Read the model definition and answer for the solid it produces. Units are mm, in the model's axes. Face numbers are marked on the shaded views. Coordinates: 2 decimals unless noted, no trailing zeros. Write each loop counter-clockwise with the first axis right and the second up, starting at its lowest first coordinate (ties: lowest second). Pieces come first, ordered by that corner, then holes. Notation, with made-up numbers: (85, 26.5) -> (141, 26.5) arc R24 ccw to (141, 44.5) -> close; hole circle Ø8 at (-29, 85.25). An arc over 180 degrees is marked (long way). Answer in a Markdown table with one row per item. Add a question column.
Item 1: For a pull along Y with two mould halves and no side action, classify the marked faces 1, 2, 3 and 4 as +Y half, -Y half, draft (parallel to the pull), parting line (faces both ways), or undercut.
Item 2: Section A-A on z = 60 is taken. Write down the section's boundary in (x, y), then the cut area to 4 significant figures.
Item 3: Straight lines are drawn through the part: line 1 (Y direction, x = 122, z = 60); line 2 (X direction, y = -77.5, z = 12); line 3 (Y direction, x = 11.5, z = 71). For each, find the intervals that lie inside material, in ascending order. Write a range as from..to.
Item 4: Given pin 1 Ø12 at (x, y) = (-84.5, 55) entering from -Z; pin 2 Ø5 at (y, z) = (52.25, 60) entering from +X, each flat-ended and moving along its own axis, determine where each tip first touches the part or whether it passes through.
Item 5: Section B-B on y = -52.25 is taken. Write down the section's boundary in (x, z).
Item 6: Section C-C on x = -53 is taken. Write down the section's boundary in (y, z), then the cut area to 3 significant figures.
Item 7: Section D-D on z = 43 is taken. Write down the section's boundary in (x, y), then the cut area to 4 significant figures.
```python
from build123d import *

# Parameters (mm, degrees)
SKIZZE1_W                       = 250
SKIZZE1_H                       = 194.5
AUFSATZ_LINEAR_AUSTRAGEN1_DEPTH = 139
SKIZZE2_W                       = 240
SKIZZE2_H                       = 184.5
SCHNITT_LINEAR_AUSTRAGEN1_DEPTH = 134
F_8_0MM_STIFTLOCH1_D            = 8


with BuildPart() as part:
    # Skizze1 → Aufsatz-Linear austragen1 (new body)
    with BuildSketch(Plane.XY):
        Rectangle(SKIZZE1_W, SKIZZE1_H)
    extrude(amount=AUFSATZ_LINEAR_AUSTRAGEN1_DEPTH)

    # Skizze2 → Schnitt-Linear austragen1 (cut)
    with BuildSketch(Plane(origin=(0, 0, 0), x_dir=(-1, 0, 0), z_dir=(0, 0, -1))):
        Rectangle(SKIZZE2_W, SKIZZE2_H)
    extrude(amount=-SCHNITT_LINEAR_AUSTRAGEN1_DEPTH, mode=Mode.SUBTRACT)

    # Ø8.0mm Stiftloch1 (through all)
    with Locations(Plane.ZY.offset(125)):
        with Locations((60, -52.25)):
            f_8_0mm_stiftloch1 = Hole(F_8_0MM_STIFTLOCH1_D / 2)

    # Spiegeln1: Ø8.0mm Stiftloch1 across plane
    add(f_8_0mm_stiftloch1.mirror(Plane.ZX), mode=Mode.SUBTRACT)


solid = part.part
```
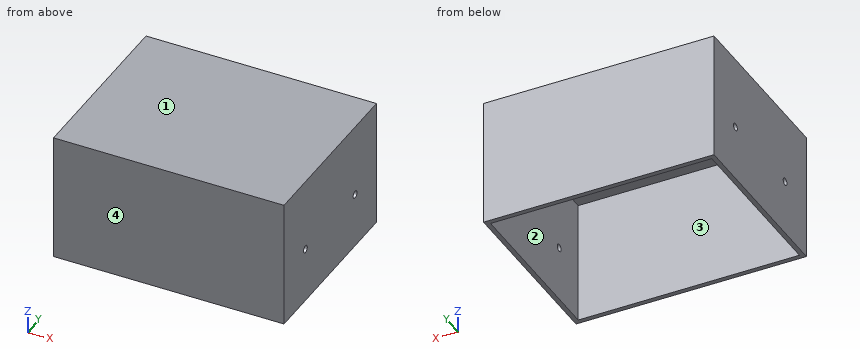
Results below:
| question | item | result |
|---|---|---|
| 1 | face 1 | draft |
| 1 | face 2 | undercut |
| 1 | face 3 | undercut |
| 1 | face 4 | -Y half |
| 2 | outline | (-125, -97.25) -> (125, -97.25) -> (125, -56.25) -> (120, -56.25) -> (120, -92.25) -> (-120, -92.25) -> (-120, -56.25) -> (-125, -56.25) -> close; (-125, -48.25) -> (-120, -48.25) -> (-120, 48.25) -> (-125, 48.25) -> close; (-125, 56.25) -> (-120, 56.25) -> (-120, 92.25) -> (120, 92.25) -> (120, 56.25) -> (125, 56.25) -> (125, 97.25) -> (-125, 97.25) -> close; (120, -48.25) -> (125, -48.25) -> (125, 48.25) -> (120, 48.25) -> close |
| 2 | area | 4,185 mm2 |
| 3 | line 1 | y = -97.25..-56.25, -48.25..48.25, 56.25..97.25 |
| 3 | line 2 | x = -125..-120, 120..125 |
| 3 | line 3 | y = -97.25..-92.25, 92.25..97.25 |
| 4 | pin 1 | stops at z = 134 |
| 4 | pin 2 | passes through |
| 5 | outline | (-125, 0) -> (-120, 0) -> (-120, 56) -> (-125, 56) -> close; (-125, 64) -> (-120, 64) -> (-120, 134) -> (120, 134) -> (120, 64) -> (125, 64) -> (125, 139) -> (-125, 139) -> close; (120, 0) -> (125, 0) -> (125, 56) -> (120, 56) -> close |
| 6 | outline | (-97.25, 0) -> (-92.25, 0) -> (-92.25, 134) -> (92.25, 134) -> (92.25, 0) -> (97.25, 0) -> (97.25, 139) -> (-97.25, 139) -> close |
| 6 | area | 2,310 mm2 |
| 7 | outline | (-125, -97.25) -> (125, -97.25) -> (125, 97.25) -> (-125, 97.25) -> close; hole (-120, -92.25) -> (120, -92.25) -> (120, 92.25) -> (-120, 92.25) -> close |
| 7 | area | 4,345 mm2 |
